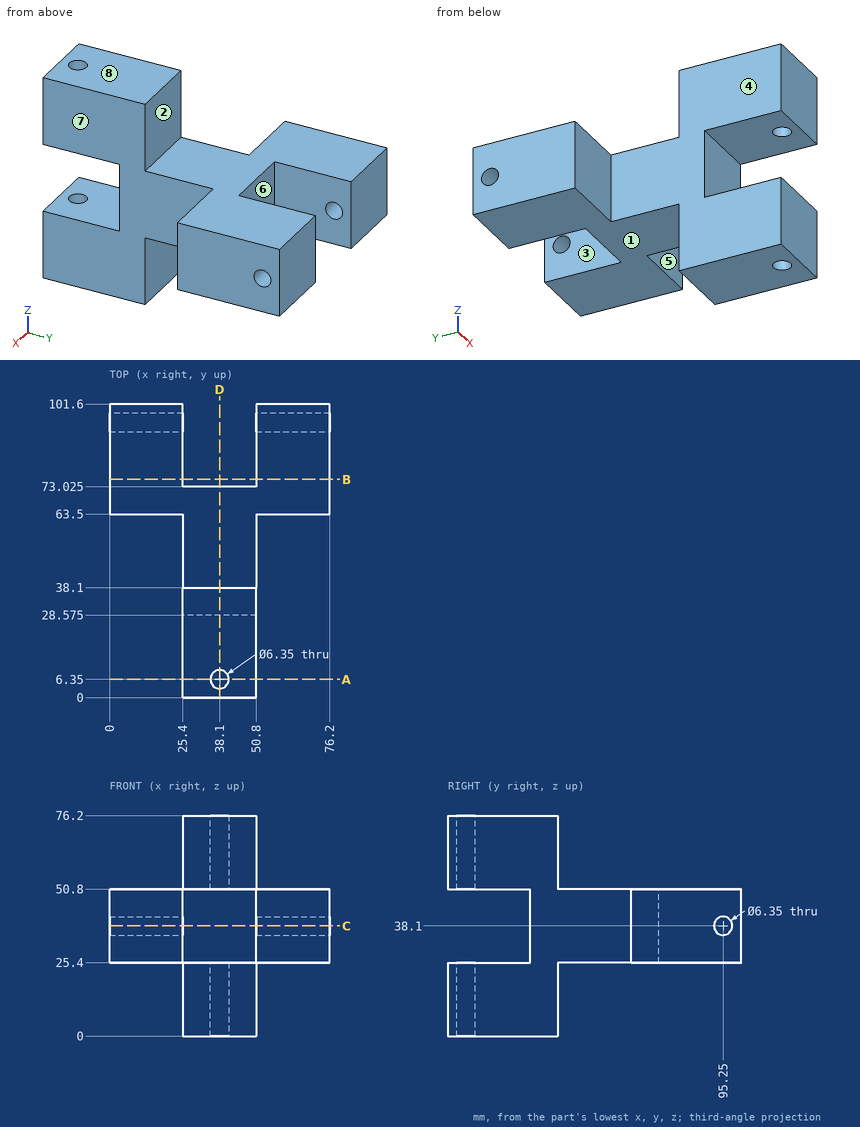
Part print with two shaded views. Sizes in mm from the minimum x, y, z corner. A direction names the side the tool comes from. Coordinates: 2 decimals unless noted, no trailing zeros. Order: outer loops, then holes, each group sorted by start corner. A loop starts at its lowest first (then second) coordinate and runs counter-clockwise, first axis right, second up.
(1) Saw through at C-C, the plane z = 38.1. Write the cut outline in (x, y) (3 decimals), and give its area (3 significant figures).
Solution:
outline: (0, 63.5) - (25.4, 63.5) - (25.4, 28.575) - (50.8, 28.575) - (50.8, 63.5) - (76.2, 63.5) - (76.2, 92.075) - (50.8, 92.075) - (50.8, 73.025) - (25.4, 73.025) - (25.4, 92.075) - (0, 92.075) - close; (0, 98.425) - (25.4, 98.425) - (25.4, 101.6) - (0, 101.6) - close; (50.8, 98.425) - (76.2, 98.425) - (76.2, 101.6) - (50.8, 101.6) - close
area: 2,740 mm2
(2) Which spindle directions (+Z, -Z, +X, -X, +Y, -Y) get a long thin tool onto all of the face, cutting with end or side? Do the marked faces 1, 2, 3, 4 and 5. Say none if no direction does.
Solution:
face 1: -Z, +X, -X, +Y
face 2: +Z, +X, -X, +Y
face 3: +Z, -Z, +Y
face 4: +Z, -Z, -X, -Y
face 5: +Z, -Z, +X, -Y
(3) Saw through at A-A, the plane y = 6.35. Write the cut outline in (x, z) (3 decimals), and give its area (3 significant figures).
Solution:
outline: (25.4, 0) - (34.925, 0) - (34.925, 25.4) - (25.4, 25.4) - close; (25.4, 50.8) - (34.925, 50.8) - (34.925, 76.2) - (25.4, 76.2) - close; (41.275, 0) - (50.8, 0) - (50.8, 25.4) - (41.275, 25.4) - close; (41.275, 50.8) - (50.8, 50.8) - (50.8, 76.2) - (41.275, 76.2) - close
area: 968 mm2
(4) Mould opens along X. For the marked faces 6, 7 and 8 say: released by +X, released by -X, zero draft, split by the parting line, or undercut.
Solution:
face 6: undercut
face 7: released by +X
face 8: zero draft
(5) Drill centre lines: L1, parallel to Z at x = 9.25, y = 95.25 (3 decimals); L2, parallel to Y at x = 38.1, z = 8.25 (3 decimals); L3, parallel to Y at x = 24, z = 47. Where is each one in solid material? Low to high.
Solution:
L1: z = 25.4 to 34.925, 41.275 to 50.8
L2: y = 0 to 3.175, 9.525 to 38.1
L3: y = 63.5 to 101.6
(6) Pin check, flat tips, straight feed: pin 1 Ø6 at (x, z) = (19.5, 41) entering from -Y; pin 2 Ø19 at (x, y) = (46.5, 73) entering from -Z; pin 3 Ø6 at (y, z) = (24.5, 64) entering from +X. Stop position of each tip, or through.
Solution:
pin 1: stops at y = 63.5
pin 2: stops at z = 25.4
pin 3: stops at x = 50.8
(7) Saw through at B-B, the plane y = 75.5. Write the cut outline in (x, z), and give its area (3 significant figures).
Solution:
outline: (0, 25.4) - (25.4, 25.4) - (25.4, 50.8) - (0, 50.8) - close; (50.8, 25.4) - (76.2, 25.4) - (76.2, 50.8) - (50.8, 50.8) - close
area: 1,290 mm2
(8) Saw through at D-D, the plane x = 38.1. Write the cut outline in (y, z) (3 decimals).
Solution:
outline: (0, 0) - (3.175, 0) - (3.175, 25.4) - (0, 25.4) - close; (0, 50.8) - (3.175, 50.8) - (3.175, 76.2) - (0, 76.2) - close; (9.525, 0) - (38.1, 0) - (38.1, 25.4) - (73.025, 25.4) - (73.025, 50.8) - (38.1, 50.8) - (38.1, 76.2) - (9.525, 76.2) - (9.525, 50.8) - (28.575, 50.8) - (28.575, 25.4) - (9.525, 25.4) - close
